The model under review builds one solid part; all positions refer to its coordinate system, in mm. A direction names the side the tool comes from. Coordinates: 2 decimals unless noted, no trailing zeros. Write each loop counter-clockwise with the first axis right and the second up, starting at its lowest first coordinate (ties: lowest second). Pieces come first, ordered by that corner, then holes. Notation, with made-up numbers: (-24, 81.25) - (-13, 81.25) arc R17 cw to (-13, 92.25) - close; hole circle Ø7 at (32, 60.5). An arc over 180 degrees is marked (long way). Return JSON: item names as keys, results as strings. Group by question number.
(1) We need section A-A on y = -20.5. State the section outline as (x, z) points (3 decimals).
(2) We need section D-D on z = -0.75. State the section outline as (x, y) points, then the cut area to 3 significant figures.
(3) Draft analysis for pull direction Y (two halves, no side actions). For faces 3 (the face through (10, -72.971, 0)), 4 (the face through (-170.16, -81.66, 0.04)), 5 (the face through (-1, -65, -3.175)), state which applies: released by +Y, released by -Y, zero draft, split by the parting line, or undercut.
(4) We need section C-C on x = -42. State the section outline as (y, z) points (3 decimals).
(5) To check wall thickness, follow L1, parallel to Y at x = -88.5, z = 2.5; L2, parallel to X at y = -22, z = 2; L3, parallel to Y at x = 145, z = 0. State the ranges of each line that lie inside material, in increasing order. Write a range as from..to.
(6) For pin 1 Ø1.9 at (y, z) = (75.5, 0) entering from +X; pin 2 Ø3 at (y, z) = (74, -0.5) entering from -X; pin 3 Ø1.9 at (x, z) = (-162.5, 0.5) entering from +Y, all flat-tipped, find the tip position at first contact; note any pin that passes through.
(7) Tool access review of faces 1 (the face through (-177.8, -1, 0)), 2 (the face through (-152.4, -1, 0)): name each direction out of +Z, -Z, +X, -X, +Y, -Y from which nothing blocks a thin tool from reaching the whole face with its end or side.
(8) We need section B-B on x = -133. State the section outline as (y, z) points (3 decimals).
```python
from build123d import *

# Parameters (mm, degrees)
F0_W      = 304.8
F0_H      = 125.8824
F1_DEPTH  = 3.175
F2_W      = 355.6
F2_H      = 177.8
F3_DEPTH  = 3.175
F4_DEPTH  = 12.7
F5_R      = 25.4
F6_R      = 25.4
F7_R      = 25.4
F8_R      = 25.4
F9_W      = 254
F9_H      = 6.35
F10_DEPTH = 12.7
F11_W     = 254
F11_H     = 6.35
F12_DEPTH = 12.7
F13_W     = 6.35
F13_H     = 101.6
F14_DEPTH = 12.7
F15_W     = 6.35
F15_H     = 101.6
F16_DEPTH = 12.7


with BuildPart() as f1:
    # F0 (on Top) → F1 (new body, symmetric)
    with BuildSketch(Plane.XY):
        Rectangle(F0_W, F0_H)
    extrude(amount=F1_DEPTH, both=True)

    # F2 (on Top) → F3 (join, symmetric)
    with BuildSketch(Plane.XY):
        Rectangle(F2_W, F2_H)
    extrude(amount=F3_DEPTH, both=True)

    # F0 (on Top) → F4 (cut, symmetric)
    with BuildSketch(Plane.XY):
        Rectangle(F0_W, F0_H)
    extrude(amount=F4_DEPTH, both=True, mode=Mode.SUBTRACT)

    # F5
    f5_edges = [f1.edges().sort_by_distance(p)[0] for p in [
        (-177.8, 88.9, 0),
    ]]
    fillet(f5_edges, radius=F5_R)

    # F6
    f6_edges = [f1.edges().sort_by_distance(p)[0] for p in [
        (177.8, 88.9, 0),
    ]]
    fillet(f6_edges, radius=F6_R)

    # F7
    f7_edges = [f1.edges().sort_by_distance(p)[0] for p in [
        (177.8, -88.9, 0),
    ]]
    fillet(f7_edges, radius=F7_R)

    # F8
    f8_edges = [f1.edges().sort_by_distance(p)[0] for p in [
        (-177.8, -88.9, 0),
    ]]
    fillet(f8_edges, radius=F8_R)

    # F9 (on face) → F10 (cut, symmetric)
    with BuildSketch(Plane.XY):
        with Locations((4.1438912572, 74.3213535368)):
            Rectangle(F9_W, F9_H)
    extrude(amount=F10_DEPTH, both=True, mode=Mode.SUBTRACT)

    # F11 (on face) → F12 (cut, symmetric)
    with BuildSketch(Plane.XY):
        with Locations((12.1505002975, -76.146347177)):
            Rectangle(F11_W, F11_H)
    extrude(amount=F12_DEPTH, both=True, mode=Mode.SUBTRACT)

    # F13 (on face) → F14 (cut, symmetric)
    with BuildSketch(Plane.XY):
        with Locations((-163.0329436541, -1.6751059711)):
            Rectangle(F13_W, F13_H)
    extrude(amount=F14_DEPTH, both=True, mode=Mode.SUBTRACT)

    # F15 (on face) → F16 (cut, symmetric)
    with BuildSketch(Plane.XY):
        with Locations((165.0233619928, 3.1901380599)):
            Rectangle(F15_W, F15_H)
    extrude(amount=F16_DEPTH, both=True, mode=Mode.SUBTRACT)


solid = f1.part
```
Ans:
{
 "1": {"outline": "(-177.8, -3.175) - (-166.208, -3.175) - (-166.208, 3.175) - (-177.8, 3.175) - close; (-159.858, -3.175) - (-152.4, -3.175) - (-152.4, 3.175) - (-159.858, 3.175) - close; (152.4, -3.175) - (161.848, -3.175) - (161.848, 3.175) - (152.4, 3.175) - close; (168.198, -3.175) - (177.8, -3.175) - (177.8, 3.175) - (168.198, 3.175) - close"},
 "2": {"outline": "(-177.8, -63.5) arc R25.4 ccw to (-152.4, -88.9) - (152.4, -88.9) arc R25.4 ccw to (177.8, -63.5) - (177.8, 63.5) arc R25.4 ccw to (152.4, 88.9) - (-152.4, 88.9) arc R25.4 ccw to (-177.8, 63.5) - close; hole (-166.21, -52.48) - (-159.86, -52.48) - (-159.86, 49.12) - (-166.21, 49.12) - close; hole (-152.4, -62.94) - (152.4, -62.94) - (152.4, 62.94) - (-152.4, 62.94) - close; hole (-122.86, 71.15) - (131.14, 71.15) - (131.14, 77.5) - (-122.86, 77.5) - close; hole (-114.85, -79.32) - (139.15, -79.32) - (139.15, -72.97) - (-114.85, -72.97) - close; hole (161.85, -47.61) - (168.2, -47.61) - (168.2, 53.99) - (161.85, 53.99) - close", "area": "19,800 mm²"},
 "3": {"face 3": "undercut", "face 4": "released by -Y", "face 5": "zero draft"},
 "4": {"outline": "(-88.9, -3.175) - (-79.321, -3.175) - (-79.321, 3.175) - (-88.9, 3.175) - close; (-72.971, -3.175) - (-62.941, -3.175) - (-62.941, 3.175) - (-72.971, 3.175) - close; (62.941, -3.175) - (71.146, -3.175) - (71.146, 3.175) - (62.941, 3.175) - close; (77.496, -3.175) - (88.9, -3.175) - (88.9, 3.175) - (77.496, 3.175) - close"},
 "5": {"L1": "-88.9..-79.32, -72.97..-62.94, 62.94..71.15, 77.5..88.9", "L2": "-177.8..-166.21, -159.86..-152.4, 152.4..161.85, 168.2..177.8", "L3": "-88.9..-62.94, 62.94..88.9"},
 "6": {"pin 1": "x = 175.27", "pin 2": "x = -176.15", "pin 3": "y = 87.19"},
 "7": {"face 1": "+Z, -Z, -X, +Y, -Y", "face 2": "+Z, -Z"},
 "8": {"outline": "(-88.9, -3.175) - (-62.941, -3.175) - (-62.941, 3.175) - (-88.9, 3.175) - close; (62.941, -3.175) - (88.9, -3.175) - (88.9, 3.175) - (62.941, 3.175) - close"}
}
